Answer from the drawing. Dimensions are ordinates in mm from the lowest x, y and z of the part. Coordinates: 2 decimals unless noted, no trailing zeros. Order: outer loops, then holes, each group sorted by start corner. A loop starts at its lowest first (then second) coordinate and runs counter-clockwise, first axis right, second up.
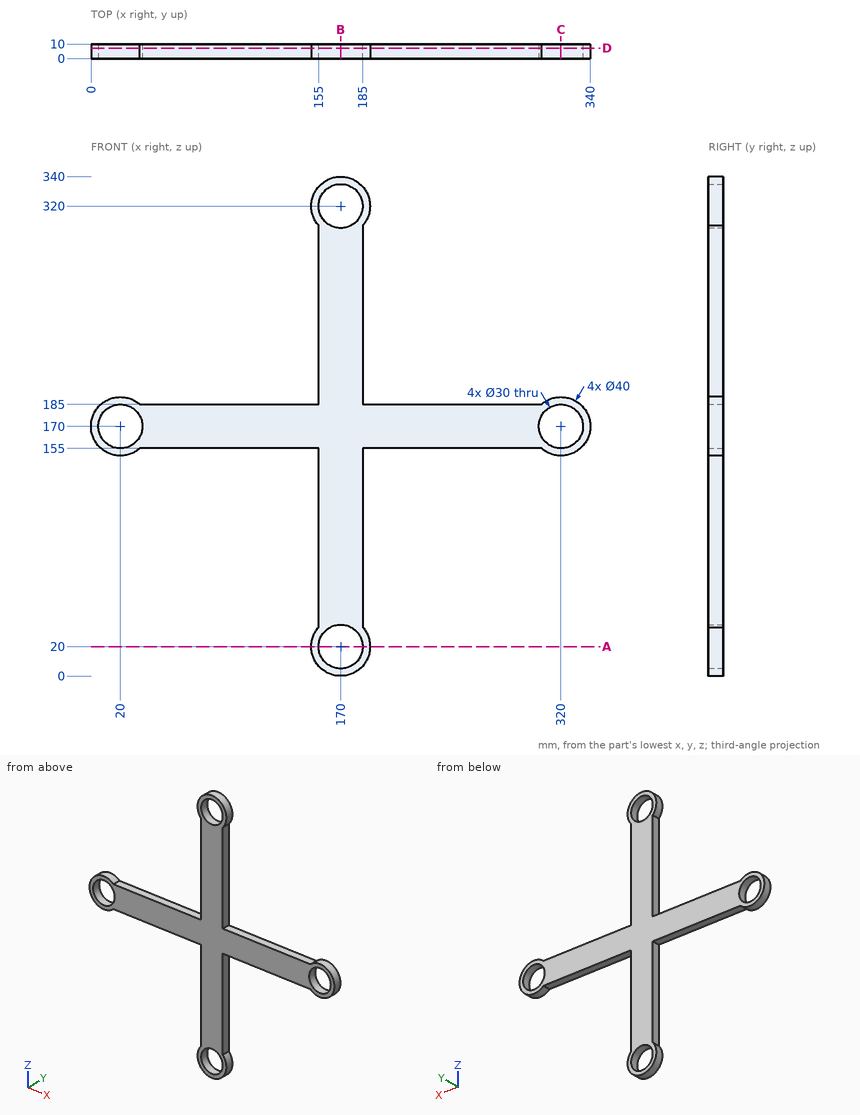
1. The part is cut by section C-C (x = 320). Determine the outline of the cut face in (y, z).
2. Consider probe 1 along Z at (x, y) = (320, 6.75); probe 2 along X at (y, z) = (6, 170). Determine where each line is inside the solid, lowest interval first.
3. Flat-ended cylindrical pins translate along their axes: pin 1 (5 mm diameter, centred on x = 250, y = 7.5, fed in from -Z); pin 2 (3 mm diameter, centred on x = 238, y = 6.5, fed in from +Z); pin 3 (3 mm diameter, centred on y = 5, z = 226.5, fed in from -X). Find the tip coordinate at first contact, or state that the pin passes through.
4. The part is cut by section A-A (z = 20). Determine the outline of the cut face in (x, y), plus the area to 4 significant figures.
5. The part is cut by section D-D (y = 7.25). Determine the outline of the cut face in (x, z), plus the area to 3 significant figures.
6. The part is cut by section B-B (x = 170). Determine the outline of the cut face in (y, z).
Worked out:
1. outline: (0, 150) - (10, 150) - (10, 155) - (0, 155) - close; (0, 185) - (10, 185) - (10, 190) - (0, 190) - close
2. probe 1: z = 150 to 155, 185 to 190
2. probe 2: x = 0 to 5, 35 to 305, 335 to 340
3. pin 1: stops at z = 155
3. pin 2: stops at z = 185
3. pin 3: stops at x = 155
4. outline: (150, 0) - (155, 0) - (155, 10) - (150, 10) - close; (185, 0) - (190, 0) - (190, 10) - (185, 10) - close
4. area: 100.0 mm2
5. outline: (33.23, 155) - (155, 155) - (155, 33.23) arc R20 ccw (long way) to (185, 33.23) - (185, 155) - (306.77, 155) arc R20 ccw (long way) to (306.77, 185) - (185, 185) - (185, 306.77) arc R20 ccw (long way) to (155, 306.77) - (155, 185) - (33.23, 185) arc R20 ccw (long way) to start; hole circle Ø30 at (20, 170); hole circle Ø30 at (170, 20); hole circle Ø30 at (170, 320); hole circle Ø30 at (320, 170)
5. area: 17,100 mm2
6. outline: (0, 0) - (10, 0) - (10, 5) - (0, 5) - close; (0, 35) - (10, 35) - (10, 305) - (0, 305) - close; (0, 335) - (10, 335) - (10, 340) - (0, 340) - close
